from build123d import *

# Parameters (mm, degrees)
SKETCH_1_W          = 114.397193433
SKETCH_1_H          = 135.669398824
EXTRUDE_1_DEPTH     = 2
SKETCH_2_R          = 4
EXTRUDE_2_DEPTH     = 39
SKETCH_3_R          = 0.9
CUT_EXTRUDE_1_DEPTH = 11
FILLET_1_R          = 10


with BuildPart() as part:
    # Эскиз1 → Бобышка-Вытянуть1 (new body)
    with BuildSketch(Plane(origin=(0, 0, 0), x_dir=(1, 0, 0), z_dir=(0, 1, 0))):
        with Locations((-0.236357837, -15.24508053)):
            Rectangle(SKETCH_1_W, SKETCH_1_H)
    extrude(amount=EXTRUDE_1_DEPTH)

    # Эскиз2 → Бобышка-Вытянуть2 (add)
    with BuildSketch(Plane(origin=(0, 2, 0), x_dir=(1, 0, 0), z_dir=(0, 1, 0))):
        with Locations((-48.434954554, 43.589618882)):
            Circle(SKETCH_2_R)
        with Locations((47.962238879, 43.589618882)):
            Circle(SKETCH_2_R)
        with Locations((47.962238879, -74.079779942)):
            Circle(SKETCH_2_R)
        with Locations((-48.434954554, -71.306708374)):
            Circle(SKETCH_2_R)
    extrude(amount=EXTRUDE_2_DEPTH)

    # Эскиз3 → Вырез-Вытянуть1 (cut)
    with BuildSketch(Plane(origin=(0, 41, 0), x_dir=(1, 0, 0), z_dir=(0, 1, 0))):
        with Locations((47.962238879, -74.079779942)):
            Circle(SKETCH_3_R)
        with Locations((-48.434954554, -71.306708374)):
            Circle(SKETCH_3_R)
        with Locations((-48.434954554, 43.589618882)):
            Circle(SKETCH_3_R)
        with Locations((47.962238879, 43.589618882)):
            Circle(SKETCH_3_R)
    extrude(amount=-CUT_EXTRUDE_1_DEPTH, mode=Mode.SUBTRACT)

    # Скругление1
    fillet_1_edges = [part.edges().sort_by_distance(p)[0] for p in [
        (-57.434954554, 1, -52.589618882),
        (56.962238879, 1, -52.589618882),
        (56.962238879, 1, 83.079779942),
        (-57.434954554, 1, 83.079779942),
    ]]
    fillet(fillet_1_edges, radius=FILLET_1_R)


solid = part.part
Verification items for the finished model (mm, model axes). A direction names the side the tool comes from. Round coordinates to 2 decimals unless told otherwise and drop trailing zeros. Loops run counter-clockwise (first coordinate to the right, second up) from the corner with the lowest first, then second, coordinate; pieces in that order, holes last. Notation, with made-up numbers: (-23.5, 0.5) - (6.5, 0.5) arc R37 ccw to (6.5, 36.5) - close; hole circle Ø3 at (29.5, 54.25). An arc over 180 degrees is marked (long way). Answer in a Markdown table with one row per item. Add a question column.
Q1. Tool access check on faces 4 (the face through (-54.583, 1.014, 80.073)), 5 (the face through (45.01, 21.23, 71.38)). Record the directions out of +Z, -Z, +X, -X, +Y, -Y that give a thin tool (end or side, any length) a straight path to the whole face; none if there is none.
Q2. Section check C-C on z = 1.5. Enter the section's corners in (x, y).
Q3. Release check for a two-part mould opening along Z. For faces 1 (the face through (-51.38, 21.23, 68.6)), 2 (the face through (-48, 41, -45)), 3 (the face through (53.955, 1.014, 80.228)) record: pulls with the +Z half, pulls with the -Z half, needs draft (parallel to the pull), parting line crosses it, or undercut.
Q4. Section check A-A on y = 38.5. Enter the section's corners in (x, z), plus the area to 3 significant figures.
Q5. Gauge pin test, flat ends, axial feed: pin 1 (2 mm diameter, centred on x = 28.5, z = -34.5, fed in from -Y); pin 2 (1 mm diameter, centred on x = 41.5, y = 21.5, fed in from +Z); pin 3 (2 mm diameter, centred on x = -33, z = 8, fed in from +Y); pin 4 (0.5 mm diameter, centred on x = 48, z = 74, fed in from +Y). Record the tip position at first contact, or that the pin passes through.
Q6. Material ranges on line 1 (Y direction, x = -37, z = -19.5); line 2 (Z direction, x = -47.5, y = 8.5); line 3 (Z direction, x = 44.5, y = 30.5), recorded low to high.
Q7. Section check B-B on x = -18.5. Enter the section's corners in (y, z), plus the area to 3 significant figures.
Q8. Section check D-D on y = 4. Enter the section's corners in (x, z).
Found:
| question | item | result |
|---|---|---|
| 1 | face 4 | +Z, -X, +Y, -Y |
| 1 | face 5 | +Y |
| 2 | outline | (-57.43, 0) - (56.96, 0) - (56.96, 2) - (-57.43, 2) - close |
| 3 | face 1 | undercut |
| 3 | face 2 | needs draft |
| 3 | face 3 | pulls with the +Z half |
| 4 | outline | circle Ø8 at (-48.43, -43.59); circle Ø8 at (-48.43, 71.31); circle Ø8 at (47.96, -43.59); circle Ø8 at (47.96, 74.08); hole circle Ø1.8 at (-48.43, -43.59); hole circle Ø1.8 at (-48.43, 71.31); hole circle Ø1.8 at (47.96, -43.59); hole circle Ø1.8 at (47.96, 74.08) |
| 4 | area | 191 mm² |
| 5 | pin 1 | stops at y = 0 |
| 5 | pin 2 | passes through |
| 5 | pin 3 | stops at y = 2 |
| 5 | pin 4 | stops at y = 30 |
| 6 | line 1 | y = 0 to 2 |
| 6 | line 2 | z = -47.48 to -39.7, 67.42 to 75.2 |
| 6 | line 3 | z = -45.59 to -41.59, 72.08 to 76.08 |
| 7 | outline | (0, -52.59) - (2, -52.59) - (2, 83.08) - (0, 83.08) - close |
| 7 | area | 271 mm² |
| 8 | outline | circle Ø8 at (-48.43, -43.59); circle Ø8 at (-48.43, 71.31); circle Ø8 at (47.96, -43.59); circle Ø8 at (47.96, 74.08) |
